from build123d import *

# Parameters (mm, degrees)
BASE_FLANGE1_DEPTH           = 2
EDGE_FLANGE1_STRIP_CUT_DEPTH = 140
EDGE_FLANGE1_DEPTH           = 140
EDGE_FLANGE2_STRIP_CUT_DEPTH = 140
EDGE_FLANGE2_DEPTH           = 140
BOSS_EXTRUDE1_DEPTH          = 2
BOSS_EXTRUDE2_START          = -2
BOSS_EXTRUDE2_DEPTH          = 2
SKETCH14_R                   = 10.1317
BOSS_EXTRUDE3_DEPTH          = 2
BOSS_EXTRUDE4_START          = -2
SKETCH15_R                   = 10.131700000000007
BOSS_EXTRUDE4_DEPTH          = 2
FILLET1_R                    = 20
SKETCH16_R                   = 3.0000000000000084
SKETCH16_R_2                 = 3.000000000000008
CUT_EXTRUDE1_DEPTH           = 116.00000000000001
BOSS_EXTRUDE5_DEPTH          = 2
BOSS_EXTRUDE6_DEPTH          = 64
BOSS_EXTRUDE8_START          = 64
BOSS_EXTRUDE8_DEPTH          = 64
SKETCH38_R                   = 3.000000000000008
SKETCH38_R_2                 = 2.9999999999999947
BOSS_EXTRUDE9_DEPTH          = 2
BOSS_EXTRUDE10_START         = -2
SKETCH40_R                   = 3.0000000000000084
BOSS_EXTRUDE10_DEPTH         = 2
CUT_EXTRUDE2_START           = -90
CUT_EXTRUDE2_DEPTH           = 90
SKETCH42_W                   = 17.233890077557817
SKETCH42_H                   = 15.447994732733191
CUT_EXTRUDE3_DEPTH           = 90
BOSS_EXTRUDE11_DEPTH         = 42.5268


# Sheet-metal steps are written as plain solids
with BuildPart() as part:
    # Sketch1 → Base-Flange1 (new body)
    with BuildSketch(Plane(origin=(0, 0, 0), x_dir=(1, 0, 0), z_dir=(0, 1, 0))):
        Polygon((69.99999999999999, 24.000000000000007), (-70.00000000000003, 23.99999999999999), (-70.00000000000003, -24.000000000000018), (69.99999999999999, -24), align=None)
    extrude(amount=-BASE_FLANGE1_DEPTH)

    # Edge-Flange1 strip (across the edge) → Edge-Flange1 strip cut (cut)
    with BuildSketch(Plane(origin=(69.99999999999999, -2, 24), x_dir=(-1.2e-16, -3.49e-15, -1), z_dir=(-1, 0, 1.2e-16))):
        Polygon((-6.736600000000024, -2.0000000000000235), (2.73660000000001, -1.9999999999999907), (2.736600000000003, 9.55e-15), (-6.736600000000031, -2.353e-14), align=None)
    extrude(amount=EDGE_FLANGE1_STRIP_CUT_DEPTH, mode=Mode.SUBTRACT)

    # Edge-Flange1 section (across the edge) → Edge-Flange1 (add)
    with BuildSketch(Plane(origin=(69.99999999999999, -2, 24), x_dir=(-1.2e-16, -3.49e-15, -1), z_dir=(-1, 0, 1.2e-16))):
        with BuildLine():
            Line((0, 0.7366000000000096), (0, 20.000000000000004))
            Line((0, 20.000000000000004), (2, 20.000000000000004))
            Line((2, 20.000000000000004), (2, 0.7366000000000096))
            ThreePointArc((2, 0.7366000000000096), (2.21574514497799, 0.21574514497799768), (2.736600000000003, 9.55e-15))
            Line((2.736600000000003, 9.55e-15), (2.73660000000001, -1.9999999999999907))
            ThreePointArc((2.73660000000001, -1.9999999999999907), (0.8015315826048977, -1.1984684173951), (0, 0.7366000000000096))
        make_face()
    extrude(amount=EDGE_FLANGE1_DEPTH)

    # Edge-Flange2 strip (across the edge) → Edge-Flange2 strip cut (cut)
    with BuildSketch(Plane(origin=(-70.00000000000003, -2, -23.999999999999993), x_dir=(1.2e-16, -3.49e-15, 1), z_dir=(1, 0, -1.2e-16))):
        Polygon((-6.736600000000024, -2.0000000000000235), (2.73660000000001, -1.9999999999999907), (2.736600000000003, 9.55e-15), (-6.736600000000031, -2.353e-14), align=None)
    extrude(amount=EDGE_FLANGE2_STRIP_CUT_DEPTH, mode=Mode.SUBTRACT)

    # Edge-Flange2 section (across the edge) → Edge-Flange2 (add)
    with BuildSketch(Plane(origin=(-70.00000000000003, -2, -23.999999999999993), x_dir=(1.2e-16, -3.49e-15, 1), z_dir=(1, 0, -1.2e-16))):
        with BuildLine():
            Line((0, 0.7366000000000096), (0, 20.000000000000004))
            Line((0, 20.000000000000004), (2, 20.000000000000004))
            Line((2, 20.000000000000004), (2, 0.7366000000000096))
            ThreePointArc((2, 0.7366000000000096), (2.21574514497799, 0.21574514497799768), (2.736600000000003, 9.55e-15))
            Line((2.736600000000003, 9.55e-15), (2.73660000000001, -1.9999999999999907))
            ThreePointArc((2.73660000000001, -1.9999999999999907), (0.8015315826048977, -1.1984684173951), (0, 0.7366000000000096))
        make_face()
    extrude(amount=EDGE_FLANGE2_DEPTH)

    # Sketch12 → Boss-Extrude1 (add)
    with BuildSketch(Plane.XY.offset(24)):
        with BuildLine():
            Line((69.99999999999997, -38.00000000000009), (69.99999999999997, -5.0936152776594525))
            Line((69.99999999999997, -5.0936152776594525), (49.99999999999997, -5.093615277659455))
            Line((49.99999999999997, -5.093615277659455), (49.99999999999997, -38.00000000000009))
            ThreePointArc((49.99999999999997, -38.00000000000009), (59.99999999999997, -48.000000000000085), (69.99999999999997, -38.00000000000009))
        make_face()
    extrude(amount=-BOSS_EXTRUDE1_DEPTH)

    # Sketch13 → Boss-Extrude2 (add)
    with BuildSketch(Plane(origin=(-2.97e-15, 8.743e-14, -23.999999999999986), x_dir=(-1, 0, 1.2e-16), z_dir=(-1.2e-16, 3.63e-15, -1)).offset(BOSS_EXTRUDE2_START)):
        with BuildLine():
            Line((-49.99999999999997, -21.999999999999922), (-49.99999999999997, -2.736599999999933))
            Line((-49.99999999999997, -2.736599999999933), (-69.99999999999999, -2.7365999999999113))
            Line((-69.99999999999999, -2.7365999999999113), (-69.99999999999997, -37.99999999999992))
            ThreePointArc((-69.99999999999997, -37.99999999999992), (-59.99999999999997, -47.999999999999915), (-49.99999999999997, -37.999999999999915))
            Line((-49.99999999999997, -37.999999999999915), (-49.99999999999997, -21.999999999999922))
        make_face()
    extrude(amount=BOSS_EXTRUDE2_DEPTH)

    # Sketch14 → Boss-Extrude3 (add)
    with BuildSketch(Plane.XY.offset(24)):
        with Locations((-70.00000000000003, -12.368300000000078)):
            Circle(SKETCH14_R)
    extrude(amount=-BOSS_EXTRUDE3_DEPTH)

    # Sketch15 → Boss-Extrude4 (add)
    with BuildSketch(Plane(origin=(-2.97e-15, 8.743e-14, -23.999999999999986), x_dir=(-1, 0, 1.2e-16), z_dir=(-1.2e-16, 3.63e-15, -1)).offset(BOSS_EXTRUDE4_START)):
        with Locations((70.00000000000003, -12.368300000000081)):
            Circle(SKETCH15_R)
    extrude(amount=BOSS_EXTRUDE4_DEPTH)

    # Fillet1
    fillet1_edges = [part.edges().sort_by_distance(p)[0] for p in [
        (49.99999999999997, -22.000000000000007, -23.000000000000075),
        (49.99999999999997, -22.000000000000007, 23.000000000000036),
    ]]
    fillet(fillet1_edges, radius=FILLET1_R)

    # Sketch16 → Cut-Extrude1 (cut)
    with BuildSketch(Plane.XY.offset(24)):
        with Locations(Location((59.99999999999997, -38.000000000000085, 0), (0, 0, 270))):
            Circle(SKETCH16_R)
        with Locations(Location((-70.00000000000003, -12.368300000000078, 0), (0, 0, 270))):
            Circle(SKETCH16_R_2)
    extrude(amount=-CUT_EXTRUDE1_DEPTH, mode=Mode.SUBTRACT)

    # Sketch23 → Boss-Extrude5 (add)
    with BuildSketch(Plane(origin=(0, 0, 0), x_dir=(1, 0, 0), z_dir=(0, 1, 0))):
        Polygon((69.99999999999999, 21.263400000000036), (149.99999999999997, 21.263400000000036), (149.99999999999997, -17.83002853781927), (149.99999999999997, -21.2634), (69.99999999999999, -21.2634), align=None)
    extrude(amount=-BOSS_EXTRUDE5_DEPTH)

    # Sketch31 → Boss-Extrude6 (add)
    with BuildSketch(Plane(origin=(69.99999999999999, 0, 0), x_dir=(0, 0, -1), z_dir=(1, 0, 0))):
        with BuildLine():
            Line((21.999999999999993, -2.736599999999998), (22.00000000000014, -37.99999999999992))
            Line((22.00000000000014, -37.99999999999992), (24.00000000000013, -37.99999999999983))
            Line((24.00000000000013, -37.99999999999983), (24, -2.736599999999978))
            ThreePointArc((24, -2.736599999999978), (23.198468417395112, -0.8015315826048983), (21.263400000000036, 0))
            Line((21.263400000000036, 0), (21.263400000000008, -2.000000000000007))
            ThreePointArc((21.263400000000008, -2.000000000000007), (21.78425485502201, -2.2157451449779955), (21.999999999999993, -2.736599999999998))
        make_face()
    extrude(amount=BOSS_EXTRUDE6_DEPTH)

    # Sketch37 → Boss-Extrude8 (add)
    with BuildSketch(Plane(origin=(69.99999999999999, 0, -8.67e-15), x_dir=(-1.2e-16, 0, -1), z_dir=(1, 0, -1.2e-16)).offset(BOSS_EXTRUDE8_START)):
        with BuildLine():
            Line((-24.000000000000007, -2.736599999999984), (-24.000000000000007, -38.00000000000001))
            Line((-24.000000000000007, -38.00000000000001), (-22.00000000000013, -38.00000000000001))
            Line((-22.00000000000013, -38.00000000000001), (-22.000000000000007, -2.736599999999991))
            ThreePointArc((-22.000000000000007, -2.736599999999991), (-21.784254855022017, -2.215745144977985), (-21.263400000000008, -2.0000000000000018))
            Line((-21.263400000000008, -2.0000000000000018), (-21.263400000000008, 0))
            ThreePointArc((-21.263400000000008, 0), (-23.198468417395112, -0.8015315826048868), (-24.000000000000007, -2.736599999999984))
        make_face()
    extrude(amount=-BOSS_EXTRUDE8_DEPTH)

    # Sketch38 → Boss-Extrude9 (add)
    with BuildSketch(Plane.XY.offset(24)):
        with BuildLine():
            ThreePointArc((-70.00000000000003, -2.2366000000000525), (-79.81974909015226, -9.873530933241609), (-74.83591228983121, -21.271406043121214))
            Line((-74.83591228983121, -21.271406043121214), (104.20534041751986, -118.52148822351042))
            ThreePointArc((104.20534041751986, -118.52148822351043), (127.65743204047538, -62.8414568179052), (133.77238644648855, -2.7342706299537234))
            Line((133.77238644648853, -2.734270629953711), (-69.95051125882394, -2.236720865704318))
            Line((-69.95051125882394, -2.236720865704318), (-70.00000000000003, -2.2366000000000574))
        make_face()
        with Locations((-70.00000000000003, -12.368300000000078)):
            Circle(SKETCH38_R, mode=Mode.SUBTRACT)
        with Locations((59.99999999999997, -38.000000000000085)):
            Circle(SKETCH38_R_2, mode=Mode.SUBTRACT)
    extrude(amount=-BOSS_EXTRUDE9_DEPTH)

    # Sketch40 → Boss-Extrude10 (add)
    with BuildSketch(Plane(origin=(-2.97e-15, 8.743e-14, -23.999999999999986), x_dir=(-1, 0, 1.2e-16), z_dir=(-1.2e-16, 3.64e-15, -1)).offset(BOSS_EXTRUDE10_START)):
        with BuildLine():
            Line((-133.99999999999997, -37.99999999999992), (-132.38333912432114, -37.99999999999992))
            ThreePointArc((-132.38333912432114, -37.99999999999992), (-122.55047625544603, -79.7501528522397), (-104.20534041751992, -118.52148822351012))
            Line((-104.20534041751992, -118.52148822351012), (74.83591228983121, -21.27140604312103))
            ThreePointArc((74.83591228983121, -21.27140604312103), (79.81974909015223, -9.873530933241451), (70.00000000000003, -2.236599999999915))
            Line((70.00000000000003, -2.236599999999915), (70.00000000000003, -2.7365999999999118))
            Line((70.00000000000003, -2.7365999999999118), (-133.99999999999997, -2.7365999999999118))
            Line((-133.99999999999997, -2.7365999999999118), (-133.99999999999997, -37.99999999999992))
        make_face()
        with Locations(Location((-59.99999999999997, -37.999999999999915, 0), (0, 0, 270))):
            Circle(SKETCH40_R, mode=Mode.SUBTRACT)
        with Locations(Location((70.00000000000003, -12.368300000000081, 0), (0, 0, 270))):
            Circle(SKETCH40_R, mode=Mode.SUBTRACT)
    extrude(amount=BOSS_EXTRUDE10_DEPTH)

    # Sketch41 → Cut-Extrude2 (cut)
    with BuildSketch(Plane(origin=(-2.97e-15, 8.743e-14, -23.999999999999986), x_dir=(-1, 0, 1.2e-16), z_dir=(-1.2e-16, 3.64e-15, -1)).offset(CUT_EXTRUDE2_START)):
        with BuildLine():
            Line((-133.99999999999991, -12.368300000000081), (-149.94232536885565, -45.23983757324427))
            Line((-149.94232536885565, -45.23983757324427), (-130.36666577541695, -50.69843495987621))
            ThreePointArc((-130.36666577541695, -50.69843495987621), (-133.08963515918902, -31.619276362446172), (-133.99999999999991, -12.368300000000081))
        make_face()
    extrude(amount=CUT_EXTRUDE2_DEPTH, mode=Mode.SUBTRACT)

    # Sketch42 → Cut-Extrude3 (cut)
    with BuildSketch(Plane(origin=(0, 0, -21.263400000000036), x_dir=(-1, 0, 0), z_dir=(0, 0, -1))):
        with Locations((-144.91808666667805, -5.115479942404007)):
            Rectangle(SKETCH42_W, SKETCH42_H)
    extrude(amount=-CUT_EXTRUDE3_DEPTH, mode=Mode.SUBTRACT)

    # Sketch43 → Boss-Extrude11 (add)
    with BuildSketch(Plane(origin=(0, 0, -21.263400000000036), x_dir=(-1, 0, 0), z_dir=(0, 0, -1))):
        with BuildLine():
            Line((-109.53531100208852, -109.78787579600389), (-111.55529945125834, -110.88396333851894))
            ThreePointArc((-111.55529945125834, -110.88396333851894), (-131.48462736674514, -57.8832164203161), (-136.27341292027893, -1.4622556169704357))
            Line((-136.27341292027893, -1.4622556169704357), (-133.93880439229082, -0.8589252153757276))
            ThreePointArc((-133.93880439229082, -0.8589252153757276), (-129.32254855641568, -57.02278781326821), (-109.53531100208852, -109.78787579600389))
        make_face()
    extrude(amount=-BOSS_EXTRUDE11_DEPTH)


solid = part.part
The listing builds one solid part. Answer for the finished solid, in the listing's coordinates (mm). A direction names the side the tool comes from. Coordinates: 2 decimals unless noted, no trailing zeros. Loops run counter-clockwise (first coordinate to the right, second up) from the corner with the lowest first, then second, coordinate; pieces in that order, holes last. Notation, with made-up numbers: (84, 16.5) -> (120, 16.5) arc R13 cw to (120, 40.5) -> close; hole circle Ø7 at (-37, -14.5). An arc over 180 degrees is marked (long way). Answer in a Markdown table with one row per item. Add a question column.
1. Flat-ended cylindrical pins translate along their axes: P1, Ø3.5, axis at x = 60, y = -38, coming from the -Z side; P2, Ø6, axis at x = -19, z = -17, coming from the -Y side; P3, Ø0.8, axis at y = -8, z = -23, coming from the +X side; P4, Ø1.4, axis at y = -1.5, z = 0, coming from the -X side. Find the tip coordinate at first contact, or state that the pin passes through.
2. The part is cut by section A-A, the plane z = -10. Write down the section's boundary in (x, y).
3. The part is cut by section D-D, the plane y = -38. Write down the section's boundary in (x, z).
4. The part is cut by section B-B, the plane y = -98. Write down the section's boundary in (x, z).
5. Consider line 1 (Z direction, x = 85, y = -94.5); line 2 (Y direction, x = 30, z = -8); line 3 (X direction, y = -38, z = 22.65). Determine where each line is inside the solid, lowest interval first. Write a range as [from, to].
6. Determine the mould class of faces 3 (the cylindrical face through (-72.93, -11.72, -22.99)), 4 (the flat face through (35, 0, 0)), 5 (the flat face through (49, -48, -24)), 6 (the cylindrical face through (126.198, -68.248, 23.014)) for opening direction Y: +Y half, -Y half, draft (parallel to the pull), parting line (faces both ways), or undercut.
7. The part is cut by section C-C, the plane x = 60. Write down the section's boundary in (y, z).
8. For faces 1 (the flat face through (52, -47, 24)), 2 (the flat face through (49, -47, -22)), determine the directions among +Z, -Z, +X, -X, +Y, -Y from which every point of the face is accessible in a straight line to the end or side of a thin tool.
Answer below:
| question | item | result |
|---|---|---|
| 1 | P1 | through |
| 1 | P2 | y = -2 |
| 1 | P3 | x = 134 |
| 1 | P4 | x = -70 |
| 2 | outline | (-70, -2) -> (134, -2) arc R204.26 cw to (109.54, -109.79) -> (111.56, -110.88) arc R206.56 ccw to (136.3, -2) -> (136.3, 0) -> (-70, 0) -> close |
| 3 | outline | (-44.04, -24) -> (57, -24) -> (57, -22) -> (-44.04, -22) -> close; (-44.04, 22) -> (57, 22) -> (57, 24) -> (-44.04, 24) -> close; (63, -24) -> (132.38, -24) -> (132.38, -22) -> (63, -22) -> close; (63, 22) -> (132.38, 22) -> (132.38, 24) -> (63, 24) -> close; (132.65, -21.26) -> (134.97, -21.26) -> (134.97, 21.26) -> (132.65, 21.26) -> close |
| 4 | outline | (66.42, -24) -> (115.16, -24) -> (115.16, -22) -> (66.42, -22) -> close; (66.42, 22) -> (115.16, 22) -> (115.16, 24) -> (66.42, 24) -> close; (115.45, -21.26) -> (117.98, -21.26) -> (117.98, 21.26) -> (115.45, 21.26) -> close |
| 5 | line 1 | [-24, -22], [22, 24] |
| 5 | line 2 | [-2, 0] |
| 5 | line 3 | [-44.04, 57], [63, 132.38] |
| 6 | face 3 | undercut |
| 6 | face 4 | +Y half |
| 6 | face 5 | draft |
| 6 | face 6 | -Y half |
| 7 | outline | (-94.51, -24) -> (-41, -24) -> (-41, -22) -> (-94.51, -22) -> close; (-94.51, 22) -> (-41, 22) -> (-41, 24) -> (-94.51, 24) -> close; (-35, -24) -> (-2.74, -24) arc R2.74 ccw to (0, -21.26) -> (0, 21.26) arc R2.74 ccw to (-2.74, 24) -> (-35, 24) -> (-35, 22) -> (-2.74, 22) arc R0.74 cw to (-2, 21.26) -> (-2, -21.26) arc R0.74 cw to (-2.74, -22) -> (-35, -22) -> close |
| 8 | face 1 | +Z, +X, -X, +Y, -Y |
| 8 | face 2 | +X, -X, -Y |
